from build123d import *

# Parameters (mm, degrees)
SKETCH1_W           = 609.6
SKETCH1_H           = 914.4
BOSS_EXTRUDE1_DEPTH = 939.8
SKETCH2_W           = 609.6
SKETCH2_H           = 304.8
BOSS_EXTRUDE2_DEPTH = 25.4
CUT_EXTRUDE1_DEPTH  = 610.6
SKETCH4_W           = 609.6
SKETCH4_H           = 609.6
BOSS_EXTRUDE3_DEPTH = 25.4
SKETCH5_W           = 609.6
SKETCH5_H           = 609.6
BOSS_EXTRUDE4_DEPTH = 558.8
SKETCH6_W           = 609.6
SKETCH6_H           = 609.6
BOSS_EXTRUDE5_DEPTH = 228.6
SKETCH7_W           = 609.6
SKETCH7_H           = 228.6
BOSS_EXTRUDE6_DEPTH = 152.4


with BuildPart() as part:
    # Sketch1 → Boss-Extrude1 (new body)
    with BuildSketch(Plane(origin=(0, 0, 0), x_dir=(1, 0, 0), z_dir=(0, 1, 0))):
        with Locations((304.8, -457.2)):
            Rectangle(SKETCH1_W, SKETCH1_H)
    extrude(amount=BOSS_EXTRUDE1_DEPTH)

    # Sketch2 → Boss-Extrude2 (add)
    with BuildSketch(Plane(origin=(0, 939.8, 0), x_dir=(1, 0, 0), z_dir=(0, 1, 0))):
        with Locations((304.8, -762)):
            Rectangle(SKETCH2_W, SKETCH2_H)
    extrude(amount=BOSS_EXTRUDE2_DEPTH)

    # Sketch3 → Cut-Extrude1 (cut, through all)
    with BuildSketch(Plane.ZY):
        Polygon((609.6, 965.2), (914.4, 939.8), (914.4, 965.2), align=None)
    extrude(amount=-CUT_EXTRUDE1_DEPTH, mode=Mode.SUBTRACT)

    # Sketch4 → Boss-Extrude3 (add)
    with BuildSketch(Plane(origin=(0, 939.8, 0), x_dir=(1, 0, 0), z_dir=(0, 1, 0))):
        with Locations((304.8, -304.8)):
            Rectangle(SKETCH4_W, SKETCH4_H)
    extrude(amount=BOSS_EXTRUDE3_DEPTH)

    # Sketch5 → Boss-Extrude4 (add)
    with BuildSketch(Plane(origin=(0, 965.2, 0), x_dir=(1, 0, 0), z_dir=(0, 1, 0))):
        with Locations((304.8, -304.8)):
            Rectangle(SKETCH5_W, SKETCH5_H)
    extrude(amount=BOSS_EXTRUDE4_DEPTH)

    # Sketch6 → Boss-Extrude5 (add)
    with BuildSketch(Plane(origin=(0, 1524, 0), x_dir=(1, 0, 0), z_dir=(0, 1, 0))):
        with Locations((304.8, -304.8)):
            Rectangle(SKETCH6_W, SKETCH6_H)
    extrude(amount=BOSS_EXTRUDE5_DEPTH)

    # Sketch7 → Boss-Extrude6 (add)
    with BuildSketch(Plane.XY.offset(609.6)):
        with Locations((304.8, 1638.3)):
            Rectangle(SKETCH7_W, SKETCH7_H)
    extrude(amount=BOSS_EXTRUDE6_DEPTH)


solid = part.part
Geometry: final body of the model. Coordinates: model frame, mm. A direction names the side the tool comes from. Round coordinates to 2 decimals unless told otherwise and drop trailing zeros. Loops run counter-clockwise (first coordinate to the right, second up) from the corner with the lowest first, then second, coordinate; pieces in that order, holes last. Notation, with made-up numbers: M -4,64 L 0,64 A20 ccw 0,102 Z; hole C 84.25,-24.5 d11. An arc over 180 degrees is marked long. Put each result on its own line as item: value. Start each with the question number.
(1) Set-up query: faces 4 (the face through (301, 1524, 685)), 5 (the face through (301, 1640, 762)), 6 (the face through (301, 0, 451)). Return all of +Z, -Z, +X, -X, +Y, -Y with unobstructed straight access to the full face (end or side cutting, diameter ignored); none if empty.
(2) Draft query along Y for faces 1 (the face through (301, 1752.6, 376)), 2 (the face through (0, 864, 451)), 3 (the face through (300.533, 952.678, 759.866)). Return one class per face: +Y half, -Y half, draft (parallel to the pull), parting line (faces both ways), or undercut.
(3) Section query C-C (z = 795). Return loops of the section in (x, y), then the cut area to 3 significant figures.
(4) Section query B-B (y = 1179). Return loops of the section in (x, z).
(5) Section query A-A (x = 425). Return loops of the section in (y, z).
(6) Material intervals for line 1 along Z through (x, y) = (122.5, 1283); line 2 along Y through (x, z) = (480.5, 715); line 3 along Z through (x, y) = (344, 1677), sorted ascending. Write a range as [from, to].
Findings below:
1. face 4: +Z, +X, -X
1. face 5: +Z, +X, -X, +Y
1. face 6: +Z, -Z, +X, -X, -Y
2. face 1: +Y half
2. face 2: draft
2. face 3: undercut
3. outline: M 0,0 L 609.6,0 L 609.6,949.75 L 0,949.75 Z
3. area: 579,000 mm2
4. outline: M 0,0 L 609.6,0 L 609.6,609.6 L 0,609.6 Z
5. outline: M 0,0 L 1752.6,0 L 1752.6,762 L 1524,762 L 1524,609.6 L 965.2,609.6 L 939.8,914.4 L 0,914.4 Z
6. line 1: z = [0, 609.6]
6. line 2: y = [0, 956.42], [1524, 1752.6]
6. line 3: z = [0, 762]
